Input: part model. Units: mm. Frame: model coordinates. Round coordinates to 2 decimals unless told otherwise and drop trailing zeros. Loops run counter-clockwise (first coordinate to the right, second up) from the corner with the lowest first, then second, coordinate; pieces in that order, holes last.
(1) Line query: line 1 (X direction, y = 1.85, z = 97); line 2 (X direction, y = 0.45, z = 99); line 3 (Z direction, x = -24, y = 0.65). Output: solid intervals per line, ascending.
(2) Cut plane C-C, the plane x = 62.5. Output: boundary loops of the cut face in (y, z).
(3) Cut plane B-B, the plane z = 93.5. Output: boundary loops of the cut face in (x, y), and give its area (3 significant figures).
(4) First-contact query: pin 1 Ø3 at (x, z) = (-53.02, 140.83) entering from -Y. Flat tip, straight axial feed; report the tip coordinate or a pass-through.
(5) Cut plane A-A, the plane y = 1.2. Give the number of separate pieces and of enclosed holes in the cut face, and give its area (3 significant figures).
from build123d import *

# Parameters (mm, degrees)
SKETCH1_R                = 1
SKETCH1_R_2              = 1.5
SKETCH1_R_3              = 1.35
MAIN_PLATE_DEPTH         = 2
SKETCH2_R                = 2.5
SCREW_HOLES_DEPTH        = 1.7
SCREW_HOLES_CHAMFER_SIZE = 1.2


with BuildPart() as part:
    # Sketch1 → Main_plate (new body)
    with BuildSketch(Plane(origin=(0, 0, 0), x_dir=(1, 0, 0), z_dir=(0, 1, 0))):
        with BuildLine():
            Line((-85.7928409, -82.301697444), (-55.755812757, -142.75024532))
            ThreePointArc((-55.755812757, -142.75024532), (-54.140343173, -144.158373046), (-52.002337011, -144.011760212))
            ThreePointArc((-52.002337011, -144.011760212), (-3.951682628, -127.514559525), (46.728283967, -123.969985789))
            Line((46.728283967, -123.969985789), (137.274321343, -129.465618584))
            ThreePointArc((137.274321343, -129.465618584), (139.300267663, -128.766971907), (140.238810242, -126.840393723))
            Line((140.238810242, -126.840393723), (146.327388064, -26.524995005))
            ThreePointArc((146.327388064, -26.524995005), (145.628741387, -24.499048684), (143.702163203, -23.560506106))
            ThreePointArc((143.702163203, -23.560506106), (94.476527457, -18.20079206), (45.987943487, -8.163512858))
            ThreePointArc((45.987943487, -8.163512858), (45.725737799, -8.109235511), (45.459546448, -8.080252452))
            Line((45.459546448, -8.080252452), (27.492609364, -6.989760902))
            ThreePointArc((27.492609364, -6.989760902), (26.515953382, -7.103440368), (25.638814565, -7.547745919))
            ThreePointArc((25.638814565, -7.547745919), (8.167641381, -16.397587105), (-11.285751241, -18.661896472))
            ThreePointArc((-11.285751241, -18.661896472), (-12.626973233, -18.913649552), (-13.689904343, -19.76947284))
            ThreePointArc((-13.689904343, -19.76947284), (-45.694454746, -53.276077835), (-84.531326007, -78.548221698))
            ThreePointArc((-84.531326007, -78.548221698), (-85.939453733, -80.163691282), (-85.7928409, -82.301697444))
        make_face()
        with Locations(Location((24.759473712, -109.793011675, 0), (0, 0, 270))):
            Circle(SKETCH1_R, mode=Mode.SUBTRACT)
        with Locations(Location((35.739268597, -110.459423178, 0), (0, 0, 270))):
            Circle(SKETCH1_R, mode=Mode.SUBTRACT)
        with Locations(Location((45.493229955, -106.563189377, 0), (0, 0, 270))):
            Circle(SKETCH1_R_2, mode=Mode.SUBTRACT)
        with Locations(Location((143.003172699, -26.823913699, 0), (0, 0, 270))):
            Circle(SKETCH1_R_3, mode=Mode.SUBTRACT)
        with Locations(Location((73.916954773, -17.899251104, 0), (0, 0, 270))):
            Circle(SKETCH1_R_3, mode=Mode.SUBTRACT)
        with Locations(Location((-11.217743895, -21.971485999, 0), (0, 0, 270))):
            Circle(SKETCH1_R_3, mode=Mode.SUBTRACT)
        with Locations(Location((-82.615354782, -81.280438678, 0), (0, 0, 270))):
            Circle(SKETCH1_R_3, mode=Mode.SUBTRACT)
        with Locations(Location((-53.022766816, -140.834565069, 0), (0, 0, 270))):
            Circle(SKETCH1_R_3, mode=Mode.SUBTRACT)
        with Locations(Location((136.975163208, -126.141388687, 0), (0, 0, 270))):
            Circle(SKETCH1_R_3, mode=Mode.SUBTRACT)
        Polygon((47.520707964, -113.598943276), (52.411707503, -113.895799309), (52.145142902, -118.287717263), (47.254143363, -117.99086123), align=None, mode=Mode.SUBTRACT)
    extrude(amount=MAIN_PLATE_DEPTH)

    # Sketch2 → Screw_holes (cut)
    with BuildSketch(Plane.XZ):
        with Locations(Location((136.975163208, 126.141388687, 0), (0, 0, 270))):
            Circle(SKETCH2_R)
        with Locations(Location((-53.022766816, 140.834565069, 0), (0, 0, 270))):
            Circle(SKETCH2_R)
        with Locations(Location((-82.615354782, 81.280438678, 0), (0, 0, 270))):
            Circle(SKETCH2_R)
        with Locations(Location((-11.217743895, 21.971485999, 0), (0, 0, 270))):
            Circle(SKETCH2_R)
        with Locations(Location((73.916954773, 17.899251104, 0), (0, 0, 270))):
            Circle(SKETCH2_R)
        with Locations(Location((143.003172699, 26.823913699, 0), (0, 0, 270))):
            Circle(SKETCH2_R)
    extrude(amount=-SCREW_HOLES_DEPTH, mode=Mode.SUBTRACT)

    # Screw_holes_chamfer
    # the kernel refuses this chamfer: 1.2 mm, written as the material it adds along each edge
    with BuildSketch(Plane(origin=(143.003172699, 1.7, 26.823913699), x_dir=(0, 0, -1), z_dir=(-1, 0, 0))) as screw_holes_chamfer_piece_1_section:
        Polygon((2.5, SCREW_HOLES_CHAMFER_SIZE), (2.5 - SCREW_HOLES_CHAMFER_SIZE, 0), (2.5, 0), align=None)
    screw_holes_chamfer_piece_1 = revolve(axis=Axis((143.003172699, 1.7, 26.823913699), (0, -1, 0)), mode=Mode.PRIVATE)
    screw_holes_chamfer_piece_1 = screw_holes_chamfer_piece_1 - Plane(origin=(143.003172699, 1.073479929, 26.823913699), x_dir=(0, 0, 1), z_dir=(0, -1, 0)) * Cylinder(1.35, 10, mode=Mode.PRIVATE)
    add(screw_holes_chamfer_piece_1)
    with BuildSketch(Plane(origin=(73.916954773, 1.7, 17.899251104), x_dir=(0, 0, -1), z_dir=(-1, 0, 0))) as screw_holes_chamfer_piece_2_section:
        Polygon((2.5, SCREW_HOLES_CHAMFER_SIZE), (2.5 - SCREW_HOLES_CHAMFER_SIZE, 0), (2.5, 0), align=None)
    screw_holes_chamfer_piece_2 = revolve(axis=Axis((73.916954773, 1.7, 17.899251104), (0, -1, 0)), mode=Mode.PRIVATE)
    screw_holes_chamfer_piece_2 = screw_holes_chamfer_piece_2 - Plane(origin=(73.916954773, 1.073479929, 17.899251104), x_dir=(0, 0, 1), z_dir=(0, -1, 0)) * Cylinder(1.35, 10, mode=Mode.PRIVATE)
    add(screw_holes_chamfer_piece_2)
    with BuildSketch(Plane(origin=(-11.217743895, 1.7, 21.971485999), x_dir=(0, 0, -1), z_dir=(-1, 0, 0))) as screw_holes_chamfer_piece_3_section:
        Polygon((2.5, SCREW_HOLES_CHAMFER_SIZE), (2.5 - SCREW_HOLES_CHAMFER_SIZE, 0), (2.5, 0), align=None)
    screw_holes_chamfer_piece_3 = revolve(axis=Axis((-11.217743895, 1.7, 21.971485999), (0, -1, 0)), mode=Mode.PRIVATE)
    screw_holes_chamfer_piece_3 = screw_holes_chamfer_piece_3 - Plane(origin=(-11.217743895, 1.073479929, 21.971485999), x_dir=(0, 0, 1), z_dir=(0, -1, 0)) * Cylinder(1.35, 10, mode=Mode.PRIVATE)
    add(screw_holes_chamfer_piece_3)
    with BuildSketch(Plane(origin=(-82.615354782, 1.7, 81.280438678), x_dir=(0, 0, -1), z_dir=(-1, 0, 0))) as screw_holes_chamfer_piece_4_section:
        Polygon((2.5, SCREW_HOLES_CHAMFER_SIZE), (2.5 - SCREW_HOLES_CHAMFER_SIZE, 0), (2.5, 0), align=None)
    screw_holes_chamfer_piece_4 = revolve(axis=Axis((-82.615354782, 1.7, 81.280438678), (0, -1, 0)), mode=Mode.PRIVATE)
    screw_holes_chamfer_piece_4 = screw_holes_chamfer_piece_4 - Plane(origin=(-82.615354782, 1.073479929, 81.280438678), x_dir=(0, 0, 1), z_dir=(0, -1, 0)) * Cylinder(1.35, 11, mode=Mode.PRIVATE)
    add(screw_holes_chamfer_piece_4)
    with BuildSketch(Plane(origin=(-53.022766816, 1.7, 140.834565069), x_dir=(0, 0, -1), z_dir=(-1, 0, 0))) as screw_holes_chamfer_piece_5_section:
        Polygon((2.5, SCREW_HOLES_CHAMFER_SIZE), (2.5 - SCREW_HOLES_CHAMFER_SIZE, 0), (2.5, 0), align=None)
    screw_holes_chamfer_piece_5 = revolve(axis=Axis((-53.022766816, 1.7, 140.834565069), (0, -1, 0)), mode=Mode.PRIVATE)
    screw_holes_chamfer_piece_5 = screw_holes_chamfer_piece_5 - Plane(origin=(-53.022766816, 1.073479929, 140.834565069), x_dir=(0, 0, 1), z_dir=(0, -1, 0)) * Cylinder(1.35, 10, mode=Mode.PRIVATE)
    add(screw_holes_chamfer_piece_5)
    with BuildSketch(Plane(origin=(136.975163208, 1.7, 126.141388687), x_dir=(0, 0, -1), z_dir=(-1, 0, 0))) as screw_holes_chamfer_piece_6_section:
        Polygon((2.5, SCREW_HOLES_CHAMFER_SIZE), (2.5 - SCREW_HOLES_CHAMFER_SIZE, 0), (2.5, 0), align=None)
    screw_holes_chamfer_piece_6 = revolve(axis=Axis((136.975163208, 1.7, 126.141388687), (0, -1, 0)), mode=Mode.PRIVATE)
    screw_holes_chamfer_piece_6 = screw_holes_chamfer_piece_6 - Plane(origin=(136.975163208, 1.073479929, 126.141388687), x_dir=(0, 0, 1), z_dir=(0, -1, 0)) * Cylinder(1.35, 10, mode=Mode.PRIVATE)
    add(screw_holes_chamfer_piece_6)

    # Sketch4 → Cut-Loft1 section 0
    with BuildSketch(Plane(origin=(-7.640186202, 0, 125.879695971), x_dir=(0.9981631713309721, 0, 0.060582863901407005), z_dir=(-0.060582863901407005, 0, 0.9981631713309721))):
        with BuildLine():
            Line((34.465569885, 10.749979768), (39.265569885, 10.749979768))
            ThreePointArc((39.265569885, 10.749979768), (44.515569885, 5.499979768), (39.265569885, 0.249979768))
            Line((39.265569885, 0.249979768), (34.465569885, 0.249979768))
            ThreePointArc((34.465569885, 0.249979768), (29.215569885, 5.499979768), (34.465569885, 10.749979768))
        make_face()
    # Sketch3 → Cut-Loft1 section 1
    with BuildSketch(Plane(origin=(-7.337271882, 0, 120.888880114), x_dir=(0.9981631713309721, 0, 0.060582863901407005), z_dir=(-0.060582863901407005, 0, 0.9981631713309721))):
        with BuildLine():
            Line((34.465569885, 9.25), (39.265569885, 9.25))
            ThreePointArc((39.265569885, 9.25), (43.015590117, 5.499979768), (39.265569885, 1.749959536))
            Line((39.265569885, 1.749959536), (34.465569885, 1.749959536))
            ThreePointArc((34.465569885, 1.749959536), (30.715549653, 5.499979768), (34.465569885, 9.25))
        make_face()
    loft(mode=Mode.SUBTRACT)


solid = part.part
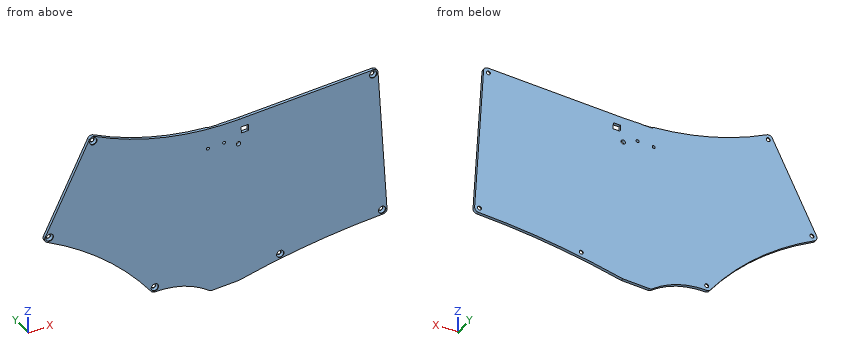
Reported:
1. line 1: x = -78.49 to 142.05
1. line 2: x = -77.5 to 141.93
1. line 3: z = 32.33 to 132.7
2. outline: (0, 12.13) - (2, 12.13) - (2, 124.93) - (0, 124.93) - close
3. outline: (-80.23, 0) - (142.26, 0) - (142.26, 2) - (-80.23, 2) - close
3. area: 445 mm2
4. pin 1: stops at y = 1.49
5. separate pieces: 1
5. enclosed holes: 10
5. area: 22,500 mm2
